Build history of the part. All positions in model axes, mm. Round coordinates to 2 decimals unless told otherwise and drop trailing zeros. Loops run counter-clockwise (first coordinate to the right, second up) from the corner with the lowest first, then second, coordinate; pieces in that order, holes last. Notation, with made-up numbers: (-29, 35) -> (11, 35) arc R31 ccw to (11, 74) -> close; hole circle Ø3 at (84.25, 82.25). An arc over 180 degrees is marked (long way). Put each result on its own line as item: value. Start each with the question number.
Item 1: Cut at C-C, the plane x = 382. List the corners of the cut face in (y, z), plus the area to 3 significant figures.
Item 2: Drill centre lines: probe 1 along X at (y, z) = (54.5, -0.5); probe 2 along Y at (x, z) = (245.5, -0.1); probe 3 along X at (y, z) = (166.5, -0.25). Where is each one in solid material? Low to high. Write a range as [from, to].
Item 3: Cut at A-A, the plane x = 68. List the corners of the cut face in (y, z).
Item 4: Cut at D-D, the plane y = 68. List the corners of the cut face in (x, z), plus the area to 3 significant figures.
Item 5: Cut at B-B, the plane y = 148. List the corners of the cut face in (x, z), plus the area to 3 significant figures.
Item 6: Flat gauge pin, fed straight in: pin 1 Ø8 at (x, y) = (9.5, 160) entering from +Z. Where does the tip first touch, or does it go through?
```python
from build123d import *

# Parameters (mm, degrees)
SKETCH1_W          = 482.6
SKETCH1_H          = 177.8
BASE_FLANGE1_DEPTH = 0.6604
SKETCH2_W          = 158.496
SKETCH2_H          = 20.574
CUT_EXTRUDE1_DEPTH = 0.6604
LPATTERN1_COUNT    = 2
LPATTERN1_PITCH    = 182.118
SKETCH3_W          = 340.614
SKETCH3_H          = 119.126
CUT_EXTRUDE2_DEPTH = 0.6604
SKETCH4_W          = 65.786
SKETCH4_H          = 152.4
CUT_EXTRUDE3_DEPTH = 0.6604
FILLET1_R          = 3.175


# Sheet-metal steps are written as plain solids
with BuildPart() as part:
    # Sketch1 → Base-Flange1 (new body)
    with BuildSketch(Plane.XY):
        with Locations((189.940791832, 97.32180564)):
            Rectangle(SKETCH1_W, SKETCH1_H)
    extrude(amount=-BASE_FLANGE1_DEPTH)

    # Sketch2 → Cut-Extrude1 (cut)
    with BuildSketch(Plane.XY):
        with Locations((59.638791832, 163.23480564)):
            Rectangle(SKETCH2_W, SKETCH2_H)
    cut_extrude1 = extrude(amount=-CUT_EXTRUDE1_DEPTH, mode=Mode.SUBTRACT)

    # LPattern1: Cut-Extrude1 ×2
    with Locations(*[(i * LPATTERN1_PITCH, 0, 0) for i in range(1, LPATTERN1_COUNT)]):
        add(cut_extrude1, mode=Mode.SUBTRACT)

    # Sketch3 → Cut-Extrude2 (cut)
    with BuildSketch(Plane.XY):
        with Locations((150.697791832, 80.68480564)):
            Rectangle(SKETCH3_W, SKETCH3_H)
    extrude(amount=-CUT_EXTRUDE2_DEPTH, mode=Mode.SUBTRACT)

    # Sketch4 → Cut-Extrude3 (cut)
    with BuildSketch(Plane(origin=(0, 0, -0.6604), x_dir=(-1, 0, 0), z_dir=(0, 0, -1))):
        with Locations((-366.597791832, 97.32180564)):
            Rectangle(SKETCH4_W, SKETCH4_H)
    extrude(amount=-CUT_EXTRUDE3_DEPTH, mode=Mode.SUBTRACT)

    # Fillet1
    fillet1_edges = [part.edges().sort_by_distance(p)[0] for p in [
        (-19.609208168, 152.94780564, -0.3302),
        (-19.609208168, 173.52180564, -0.3302),
        (138.886791832, 173.52180564, -0.3302),
        (138.886791832, 152.94780564, -0.3302),
        (162.508791832, 152.94780564, -0.3302),
        (162.508791832, 173.52180564, -0.3302),
        (321.004791832, 173.52180564, -0.3302),
        (321.004791832, 152.94780564, -0.3302),
        (-19.609208168, 21.12180564, -0.3302),
        (-19.609208168, 140.24780564, -0.3302),
        (321.004791832, 140.24780564, -0.3302),
        (321.004791832, 21.12180564, -0.3302),
        (399.490791832, 21.12180564, -0.3302),
        (399.490791832, 173.52180564, -0.3302),
        (333.704791832, 173.52180564, -0.3302),
        (333.704791832, 21.12180564, -0.3302),
    ]]
    fillet(fillet1_edges, radius=FILLET1_R)


solid = part.part
```
Reply:
1. outline: (8.42, -0.66) -> (21.12, -0.66) -> (21.12, 0) -> (8.42, 0) -> close; (173.52, -0.66) -> (186.22, -0.66) -> (186.22, 0) -> (173.52, 0) -> close
1. area: 16.8 mm^2
2. probe 1: x = [-51.36, -19.61], [321, 333.7], [399.49, 431.24]
2. probe 2: y = [8.42, 21.12], [140.25, 152.95], [173.52, 186.22]
2. probe 3: x = [-51.36, -19.61], [138.89, 162.51], [321, 333.7], [399.49, 431.24]
3. outline: (8.42, -0.66) -> (21.12, -0.66) -> (21.12, 0) -> (8.42, 0) -> close; (140.25, -0.66) -> (152.95, -0.66) -> (152.95, 0) -> (140.25, 0) -> close; (173.52, -0.66) -> (186.22, -0.66) -> (186.22, 0) -> (173.52, 0) -> close
4. outline: (-51.36, -0.66) -> (-19.61, -0.66) -> (-19.61, 0) -> (-51.36, 0) -> close; (321, -0.66) -> (333.7, -0.66) -> (333.7, 0) -> (321, 0) -> close; (399.49, -0.66) -> (431.24, -0.66) -> (431.24, 0) -> (399.49, 0) -> close
4. area: 50.3 mm^2
5. outline: (-51.36, -0.66) -> (333.7, -0.66) -> (333.7, 0) -> (-51.36, 0) -> close; (399.49, -0.66) -> (431.24, -0.66) -> (431.24, 0) -> (399.49, 0) -> close
5. area: 275 mm^2
6. pin 1: passes through
